from build123d import *

# Parameters (mm, degrees)
BOSS_EXTRUDE1_DEPTH = 2
BOSS_EXTRUDE2_DEPTH = 0.2


with BuildPart() as part:
    # Sketch1 → Boss-Extrude1 (new body)
    with BuildSketch(Plane.XY):
        with BuildLine():
            Line((-7.25, 6.9), (-7.25, 5.9))
            ThreePointArc((-7.25, 5.9), (-5.45, 0), (-7.25, -5.9))
            Line((-7.25, -5.9), (-7.25, -6.9))
            Line((-7.25, -6.9), (7.25, -6.9))
            Line((7.25, -6.9), (7.25, 6.9))
            Line((7.25, 6.9), (-7.25, 6.9))
        make_face()
        with BuildLine():
            Line((-3.75, -4.5), (-3.75, 4.5))
            ThreePointArc((-3.75, 4.5), (-2.75, 5.5), (-1.75, 4.5))
            Line((-1.75, 4.5), (-1.75, -4.5))
            ThreePointArc((-1.75, -4.5), (-2.75, -5.5), (-3.75, -4.5))
        make_face(mode=Mode.SUBTRACT)
    extrude(amount=BOSS_EXTRUDE1_DEPTH)

    # Sketch2 → Boss-Extrude2 (add)
    with BuildSketch(Plane.XY):
        with BuildLine():
            Line((-5.15, 7.25), (-5.35, 7.25))
            Line((-5.35, 7.25), (-5.35, 6.9))
            Line((-5.35, 6.9), (-4.15, 6.9))
            Line((-4.15, 6.9), (-4.15, 7.25))
            Line((-4.15, 7.25), (-4.35, 7.25))
            ThreePointArc((-4.35, 7.25), (-4.75, 7.05), (-5.15, 7.25))
        make_face()
        with BuildLine():
            Line((2.65, 7.25), (2.85, 7.25))
            ThreePointArc((2.85, 7.25), (3.25, 7.05), (3.65, 7.25))
            Line((3.65, 7.25), (3.85, 7.25))
            Line((3.85, 7.25), (3.85, 6.9))
            Line((3.85, 6.9), (2.65, 6.9))
            Line((2.65, 6.9), (2.65, 7.25))
        make_face()
        with BuildLine():
            Line((3.65, -7.25), (3.85, -7.25))
            Line((3.85, -7.25), (3.85, -6.9))
            Line((3.85, -6.9), (2.65, -6.9))
            Line((2.65, -6.9), (2.65, -7.25))
            Line((2.65, -7.25), (2.85, -7.25))
            ThreePointArc((2.85, -7.25), (3.25, -7.05), (3.65, -7.25))
        make_face()
        with BuildLine():
            Line((-4.15, -7.25), (-4.35, -7.25))
            ThreePointArc((-4.35, -7.25), (-4.75, -7.05), (-5.15, -7.25))
            Line((-5.15, -7.25), (-5.35, -7.25))
            Line((-5.35, -7.25), (-5.35, -6.9))
            Line((-5.35, -6.9), (-4.15, -6.9))
            Line((-4.15, -6.9), (-4.15, -7.25))
        make_face()
    extrude(amount=BOSS_EXTRUDE2_DEPTH)


solid = part.part
Verification items for the finished model (mm, model axes). A direction names the side the tool comes from. Coordinates: 2 decimals unless noted, no trailing zeros. Write each loop counter-clockwise with the first axis right and the second up, starting at its lowest first coordinate (ties: lowest second). Pieces come first, ordered by that corner, then holes. Notation, with made-up numbers: (-8, -34) -> (16, -34) arc R21 cw to (16, 0) -> close; hole circle Ø8 at (39, 7). An arc over 180 degrees is marked (long way). One line per item, written item: value. Start each with the question number.
Q1. Go/stop test with a flat-tipped pin: P1, Ø0.6, axis at x = 2.5, z = 0.5, coming from the +Y side. Record where the tip stops, or that it passes through.
Q2. Thickness scan on L1, parallel to X at y = -0.25, z = 1.1; L2, parallel to Y at x = -1, z = 1.6; L3, parallel to X at y = 2.25, z = 1.85. Record the ranges inside material, lowest first. Write a range as from..to.
Q3. Cross-section at C-C on x = 1. Enter the section's corners in (y, z).
Q4. Cross-section at A-A on x = -2.75. Enter the section's corners in (y, z).
Q5. Mould release check, pull along Y, two halves, no side actions. Record for faces 1 (the flat face through (2, 0, 2)), 2 (the cylindrical face through (-2.7, -5.5, 1)): pulls with the +Y half, pulls with the -Y half, needs draft (parallel to the pull), parting line crosses it, or undercut.
Q6. Cross-section at B-B on y = 3. Enter the section's corners in (x, z).
Q7. Access from +Z, -Z, +X, -X, +Y, -Y to the whole of each face (thin tool, end or side, straight path). Record for faces 3 (the flat face through (-7.25, -6.4, 1)), 4 (the flat face through (-1.75, 0, 1)).
Checked values:
1. P1: stops at y = 6.9
2. L1: x = -5.45..-3.75, -1.75..7.25
2. L2: y = -6.9..6.9
2. L3: x = -5.69..-3.75, -1.75..7.25
3. outline: (-6.9, 0) -> (6.9, 0) -> (6.9, 2) -> (-6.9, 2) -> close
4. outline: (-6.9, 0) -> (-5.5, 0) -> (-5.5, 2) -> (-6.9, 2) -> close; (5.5, 0) -> (6.9, 0) -> (6.9, 2) -> (5.5, 2) -> close
5. face 1: needs draft
5. face 2: undercut
6. outline: (-5.88, 0) -> (-3.75, 0) -> (-3.75, 2) -> (-5.88, 2) -> close; (-1.75, 0) -> (7.25, 0) -> (7.25, 2) -> (-1.75, 2) -> close
7. face 3: +Z, -Z, -X, +Y, -Y
7. face 4: +Z, -Z
